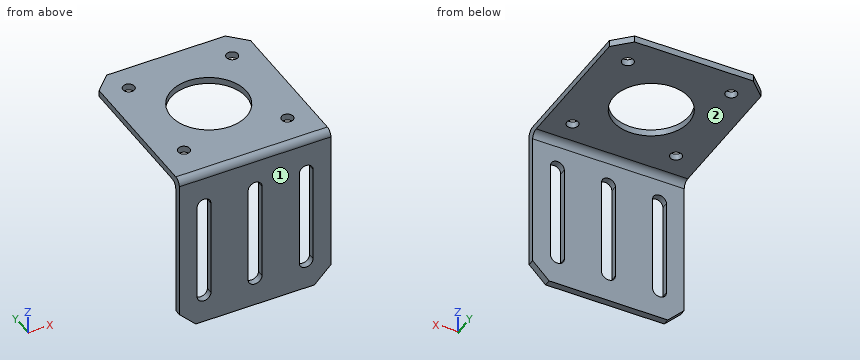
```python
from build123d import *

# Parameters (mm, degrees)
SALIENTE_EXTRUIR1_DEPTH = 46
CROQUIS2_R              = 11.5
CROQUIS2_R_2            = 1.75
CORTAR_EXTRUIR1_DEPTH   = 85.356386836
CORTAR_EXTRUIR2_DEPTH   = 85.356386836
CHAFL_N1_SIZE           = 5
CORTE_EXTRUS_O1_DEPTH   = 85.356386836


with BuildPart() as part:
    # Croquis1 → Saliente-Extruir1 (new body)
    with BuildSketch(Plane(origin=(0, 0, 0), x_dir=(0, 0, -1), z_dir=(1, 0, 0))):
        with BuildLine():
            Line((2, 0), (50, 0))
            Line((50, 0), (50, 2))
            Line((50, 2), (4, 2))
            ThreePointArc((4, 2), (2.585786438, 2.585786438), (2, 4))
            Line((2, 4), (2, 50))
            Line((2, 50), (0, 50))
            Line((0, 50), (0, 2))
            ThreePointArc((0, 2), (0.585786438, 0.585786438), (2, 0))
        make_face()
    extrude(amount=SALIENTE_EXTRUIR1_DEPTH)

    # Croquis2 → Cortar-Extruir1 (cut, through all)
    with BuildSketch(Plane.XY):
        with Locations((23, 26)):
            Circle(CROQUIS2_R)
        with Locations((7.5, 42.25)):
            Circle(CROQUIS2_R_2)
        with Locations((38.5, 41.5)):
            Circle(CROQUIS2_R_2)
        with Locations((7.5, 11.25)):
            Circle(CROQUIS2_R_2)
        with Locations((38.5, 10.5)):
            Circle(CROQUIS2_R_2)
    extrude(amount=-CORTAR_EXTRUIR1_DEPTH, mode=Mode.SUBTRACT)

    # Croquis3 → Cortar-Extruir2 (cut, through all)
    with BuildSketch(Plane.XZ):
        with BuildLine():
            Line((5.4, -11), (5.4, -41))
            ThreePointArc((5.4, -41), (7.5, -43.1), (9.6, -41))
            Line((9.6, -41), (9.6, -11))
            ThreePointArc((9.6, -11), (7.5, -8.9), (5.4, -11))
        make_face()
        with BuildLine():
            Line((36.4, -11), (36.4, -41))
            ThreePointArc((36.4, -41), (38.5, -43.1), (40.6, -41))
            Line((40.6, -41), (40.6, -11))
            ThreePointArc((40.6, -11), (38.5, -8.9), (36.4, -11))
        make_face()
    extrude(amount=-CORTAR_EXTRUIR2_DEPTH, mode=Mode.SUBTRACT)

    # Chaflán1
    chafl_n1_edges = [part.edges().sort_by_distance(p)[0] for p in [
        (0, 1, -50),
        (46, 50, -1),
        (46, 1, -50),
        (0, 50, -1),
    ]]
    chamfer(chafl_n1_edges, length=CHAFL_N1_SIZE)

    # Esboço1 → Corte-extrusão1 (cut, through all)
    with BuildSketch(Plane.XZ):
        with BuildLine():
            Line((20.9, -41), (20.9, -11))
            ThreePointArc((20.9, -11), (23, -8.9), (25.1, -11))
            Line((25.1, -11), (25.1, -41))
            ThreePointArc((25.1, -41), (23, -43.1), (20.9, -41))
        make_face()
    extrude(amount=-CORTE_EXTRUS_O1_DEPTH, mode=Mode.SUBTRACT)


solid = part.part
```
Work out the finished part from the listing and answer in its coordinate system (mm). Face numbers are marked on the shaded views. A direction names the side the tool comes from. Give positions to 0.01 mm unless a question says otherwise; leave off trailing zeros. Loops run counter-clockwise (first coordinate to the right, second up) from the corner with the lowest first, then second, coordinate; pieces in that order, holes last. Notation, with made-up numbers: (65.5, -13.75) -> (72.5, -13.75) arc R20 ccw to (72.5, 24.25) -> close; hole circle Ø1 at (4, 43.5). An arc over 180 degrees is marked (long way). Put each result on its own line as item: value. Start each with the question number.
Item 1: Each of these flat-tipped pins is pushed along its axis until it touches: P1, Ø3, axis at x = 35, y = 28, coming from the -Z side; P2, Ø8, axis at x = 9, z = -28.5, coming from the +Y side. Where does it stop, or does it pass through?
Item 2: The part is cut by section B-B (y = 26). Give the vertices of the cut face in (x, z), then the cut area to 3 significant figures.
Item 3: Which of the six approach directions +Z, -Z, +X, -X, +Y, -Y give full straight-line access (tool end or side, diameter ignored) to the marked faces 1 and 2?
Item 4: The part is cut by section A-A (x = 7.5). Give the vertices of the cut face in (y, z), then the cut area to 3 significant figures.
Item 5: The part is cut by section D-D (x = 31.5). Give the vertices of the cut face in (y, z).
Item 6: Find the intervals of material crossed by L1, parallel to Y at x = 7.5, z = -1.45; L2, parallel to Y at x = 38.5, z = -1.25; L3, parallel to Y at x = 6, z = -46, in increasing order. Write a range as [from, to].
Item 7: The part is cut by section C-C (z = -23). Give the vertices of the cut face in (x, y), then the cut area to 3 significant figures.
Answers below:
1. P1: z = -2
1. P2: y = 2
2. outline: (0, -2) -> (11.5, -2) -> (11.5, 0) -> (0, 0) -> close; (34.5, -2) -> (46, -2) -> (46, 0) -> (34.5, 0) -> close
2. area: 46.0 mm2
3. face 1: +Z, -Z, +X, -X, -Y
3. face 2: -Z, +X, -X, +Y
4. outline: (0, -50) -> (2, -50) -> (2, -43.1) -> (0, -43.1) -> close; (0, -8.9) -> (2, -8.9) -> (2, -4) arc R2 cw to (4, -2) -> (9.5, -2) -> (9.5, 0) -> (2, 0) arc R2 ccw to (0, -2) -> close; (13, -2) -> (40.5, -2) -> (40.5, 0) -> (13, 0) -> close; (44, -2) -> (50, -2) -> (50, 0) -> (44, 0) -> close
4. area: 114 mm2
5. outline: (0, -50) -> (2, -50) -> (2, -4) arc R2 cw to (4, -2) -> (18.25, -2) -> (18.25, 0) -> (2, 0) arc R2 ccw to (0, -2) -> close; (33.75, -2) -> (50, -2) -> (50, 0) -> (33.75, 0) -> close
6. L1: [0.08, 9.5], [13, 40.5], [44, 50]
6. L2: [0.15, 8.75], [12.25, 39.75], [43.25, 50]
6. L3: [0, 2]
7. outline: (0, 0) -> (5.4, 0) -> (5.4, 2) -> (0, 2) -> close; (9.6, 0) -> (20.9, 0) -> (20.9, 2) -> (9.6, 2) -> close; (25.1, 0) -> (36.4, 0) -> (36.4, 2) -> (25.1, 2) -> close; (40.6, 0) -> (46, 0) -> (46, 2) -> (40.6, 2) -> close
7. area: 66.8 mm2
